The figure shows three views and two pictorial views of one solid part (mm, origin at its lowest corner). Answer the questions. A direction names the side the tool comes from. Give positions to 0.01 mm unless a question says otherwise; leave off trailing zeros. Write each loop counter-clockwise with the first axis right and the second up, starting at its lowest first coordinate (ties: lowest second). Pieces come first, ordered by that corner, then holes. Notation, with made-up numbers: (-24.5, -17.75) -> (21.5, -17.75) arc R15 cw to (21.5, -5.75) -> close; hole circle Ø7 at (60, 60.25). An arc over 180 degrees is marked (long way). Answer as CSV lines item,"result". Start each with the question number.
1. Find the intervals of material crossed by line 1 (Z direction, x = 54, y = 102.5); line 2 (Y direction, x = 47, z = 12.25); line 3 (Y direction, x = 34, z = 24), in increasing order.
2. The part is cut by section B-B, the plane x = 65. Determine the outline of the cut face in (y, z).
3. The part is cut by section A-A, the plane y = 62.5. Determine the outline of the cut face in (x, z).
4. The part is cut by section D-D, the plane y = 127. Determine the outline of the cut face in (x, z).
5. A tool of negligible diameter and unlimited length cuts with its end or side. For the marked faces 1 and 2, from which of +Z, -Z, +X, -X, +Y, -Y can it reach the whole face along a straight path? Write none if from no direction.
6. Given pin 1 (10 mm diameter, centred on y = 113.5, z = 14, fed in from -X); pin 2 (5 mm diameter, centred on x = 62.5, y = 25.5, fed in from +Z); pin 3 (4 mm diameter, centred on x = 23.5, z = 5, fed in from -Y), each flat-ended and moving along its own axis, determine where each tip first touches the part or whether it passes through.
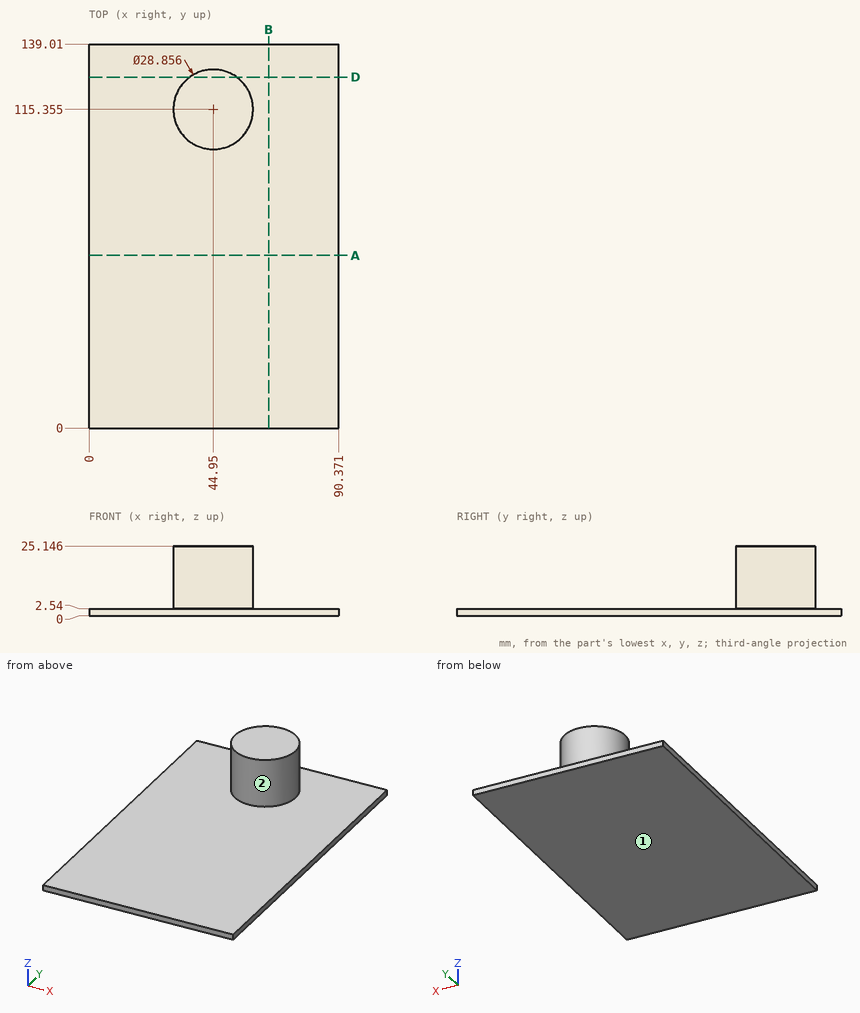
Results found:
1,line 1,"z = 0 to 2.54"
1,line 2,"y = 101.07 to 129.64"
1,line 3,"y = 105.96 to 124.75"
2,outline,"(0, 0) -> (139.01, 0) -> (139.01, 2.54) -> (0, 2.54) -> close"
3,outline,"(0, 0) -> (90.37, 0) -> (90.37, 2.54) -> (0, 2.54) -> close"
4,outline,"(0, 0) -> (90.37, 0) -> (90.37, 2.54) -> (53.47, 2.54) -> (53.47, 25.15) -> (36.43, 25.15) -> (36.43, 2.54) -> (0, 2.54) -> close"
5,face 1,"-Z, +X, -X, +Y, -Y"
5,face 2,"+Z"
6,pin 1,"stops at x = 30.52"
6,pin 2,"stops at z = 2.54"
6,pin 3,"passes through"
